Input: part model. Units: mm. Frame: model coordinates. A direction names the side the tool comes from. Round coordinates to 2 decimals unless told otherwise and drop trailing zeros. Order: outer loops, then holes, each group sorted by start corner. A loop starts at its lowest first (then second) coordinate and runs counter-clockwise, first axis right, second up. Notation, with made-up numbers: (-4, -18.75) -> (36, -18.75) arc R16 cw to (36, -5.75) -> close; hole circle Ø7 at (2.25, 80). An arc over 180 degrees is marked (long way). Use a Markdown table: item, result.
from build123d import *

# Parameters (mm, degrees)
CYLINDER_R             = 2.4
CYLINDER_DEPTH         = 10
CYLINDER_ROLL_ANGLE    = 90
CYLINDER001_R          = 8
CYLINDER001_DEPTH      = 2
CYLINDER001_ROLL_ANGLE = 90


with BuildPart() as obj1:
    # Cylinder → Cylinder (new body)
    with BuildSketch(Plane.XY):
        Circle(CYLINDER_R)
    extrude(amount=CYLINDER_DEPTH)


with BuildPart() as obj1_1:
    # Cylinder roll: moved
    add(obj1.part.rotate(Axis((0, 0, 0), (1, 0, 0)), CYLINDER_ROLL_ANGLE))


with BuildPart() as obj1_2:
    # Cylinder placement: moved
    add(obj1_1.part)


with BuildPart() as pivot:
    # Cylinder001 → Cylinder001 (new body)
    with BuildSketch(Plane.XY):
        Circle(CYLINDER001_R)
    extrude(amount=CYLINDER001_DEPTH)


with BuildPart() as pivot_1:
    # Cylinder001 roll: moved
    add(pivot.part.rotate(Axis((0, 0, 0), (1, 0, 0)), CYLINDER001_ROLL_ANGLE))


with BuildPart() as pivot_2:
    # Cylinder001 placement: moved
    add(pivot_1.part)

    # Fusion002: union obj1
    add(obj1_2.part)


solid = pivot_2.part
1) Cut plane C-C on y = -6. Return loops of the section in (x, z).
Results found:
| item | result |
|---|---|
| outline | circle Ø4.8 at (0, 0) |
2) Cut plane D-D on z = 3.75. Return loops of the section in (x, y).
Results found:
| item | result |
|---|---|
| outline | (-7.07, -2) -> (7.07, -2) -> (7.07, 0) -> (-7.07, 0) -> close |
3) Pin query (flat end, axial travel): pin 1 Ø1.5 at (x, y) = (-1.5, -4.5) entering from +Z; pin 2 Ø1 at (x, y) = (-4, -5.5) entering from +Z; pin 3 Ø1.5 at (y, z) = (-1.5, 4.5) entering from +X; pin 4 Ø1.5 at (y, z) = (-1.5, 6.5) entering from +X. Return the tip coordinate at first contact, or that it passes through.
Results found:
| item | result |
|---|---|
| pin 1 | stops at z = 2.28 |
| pin 2 | passes through |
| pin 3 | stops at x = 7.07 |
| pin 4 | stops at x = 5.56 |
4) Set-up query: faces 1 (the flat face through (0, -10, 0)), 2 (the flat face through (2, -2, 2)). Return all of +Z, -Z, +X, -X, +Y, -Y with unobstructed straight access to the full face (end or side cutting, diameter ignored); none if empty.
Results found:
| item | result |
|---|---|
| face 1 | +Z, -Z, +X, -X, -Y |
| face 2 | -Y |
5) Cut plane A-A on x = 0. Return loops of the section in (y, z).
Results found:
| item | result |
|---|---|
| outline | (-10, -2.4) -> (-2, -2.4) -> (-2, -8) -> (0, -8) -> (0, 8) -> (-2, 8) -> (-2, 2.4) -> (-10, 2.4) -> close |
6) Line query: L1, parallel to Y at x = 4, z = -0.5; L2, parallel to X at y = -6, z = -1.5; L3, parallel to X at y = -0.5, z = 5 (3 decimals). Output: solid intervals per line, ascending. Write a range as [from, to].
Results found:
| item | result |
|---|---|
| L1 | y = [-2, 0] |
| L2 | x = [-1.87, 1.87] |
| L3 | x = [-6.245, 6.245] |
7) Cut plane B-B on z = 0. Return loops of the section in (x, y), and give its area (3 significant figures).
Results found:
| item | result |
|---|---|
| outline | (-8, -2) -> (-2.4, -2) -> (-2.4, -10) -> (2.4, -10) -> (2.4, -2) -> (8, -2) -> (8, 0) -> (-8, 0) -> close |
| area | 70.4 mm² |
